```python
from build123d import *

# Parameters (mm, degrees)
SKETCH1_R           = 4.5
BOSS_EXTRUDE1_DEPTH = 8
SKETCH2_W           = 10
SKETCH2_H           = 25
BOSS_EXTRUDE2_DEPTH = 34.4
SKETCH5_W           = 10
SKETCH5_H           = 10
BOSS_EXTRUDE4_DEPTH = 8
SKETCH6_R           = 1.5
CUT_EXTRUDE1_DEPTH  = 15
SKETCH10_W          = 25
SKETCH10_H          = 32.5
BOSS_EXTRUDE6_DEPTH = 12
SKETCH12_W          = 12
SKETCH12_H          = 21.5
CUT_EXTRUDE3_DEPTH  = 21.5
SKETCH13_R          = 1
CUT_EXTRUDE4_DEPTH  = 10
SKETCH14_W          = 9
SKETCH14_H          = 13
CUT_EXTRUDE5_DEPTH  = 38.45
CUT_EXTRUDE6_REACH  = 59
SKETCH15_W          = 15
SKETCH15_H          = 20.5
SKETCH16_R          = 3
BOSS_EXTRUDE7_DEPTH = 5


with BuildPart() as part:
    # Sketch1 → Boss-Extrude1 (new body)
    with BuildSketch(Plane(origin=(0, 0, 0), x_dir=(1, 0, 0), z_dir=(0, 1, 0))):
        with BuildLine():
            Line((0, 0), (40, 0))
            ThreePointArc((40, 0), (43.535533906, 1.464466094), (45, 5))
            Line((45, 5), (45, 20))
            ThreePointArc((45, 20), (43.535533906, 23.535533906), (40, 25))
            Line((40, 25), (0, 25))
            Line((0, 25), (0, 0))
        make_face()
        with Locations((37.263316161, 12.5)):
            Circle(SKETCH1_R, mode=Mode.SUBTRACT)
    extrude(amount=BOSS_EXTRUDE1_DEPTH)

    # Sketch2 → Boss-Extrude2 (add)
    with BuildSketch(Plane(origin=(0, 8, 0), x_dir=(1, 0, 0), z_dir=(0, 1, 0))):
        with Locations((5, 12.5)):
            Rectangle(SKETCH2_W, SKETCH2_H)
    extrude(amount=BOSS_EXTRUDE2_DEPTH)

    # Sketch5 → Boss-Extrude4 (add)
    with BuildSketch(Plane(origin=(0, 42.4, 0), x_dir=(1, 0, 0), z_dir=(0, 1, 0))):
        with Locations((5, 12.5)):
            Rectangle(SKETCH5_W, SKETCH5_H)
    extrude(amount=BOSS_EXTRUDE4_DEPTH)

    # Sketch6 → Cut-Extrude1 (cut)
    with BuildSketch(Plane(origin=(0, 42.4, 0), x_dir=(1, 0, 0), z_dir=(0, 1, 0))):
        with Locations((5, 21.25)):
            Circle(SKETCH6_R)
        with Locations((5, 3.75)):
            Circle(SKETCH6_R)
    extrude(amount=-CUT_EXTRUDE1_DEPTH, mode=Mode.SUBTRACT)

    # Sketch10 → Boss-Extrude6 (add)
    with BuildSketch(Plane.ZY):
        with Locations((-12.5, 21.2)):
            Rectangle(SKETCH10_W, SKETCH10_H)
    extrude(amount=BOSS_EXTRUDE6_DEPTH)

    # Sketch12 → Cut-Extrude3 (cut)
    with BuildSketch(Plane(origin=(0, 0, -25), x_dir=(-1, 0, 0), z_dir=(0, 0, -1))):
        with Locations((3, 21.2)):
            Rectangle(SKETCH12_W, SKETCH12_H)
    extrude(amount=-CUT_EXTRUDE3_DEPTH, mode=Mode.SUBTRACT)

    # Sketch13 → Cut-Extrude4 (cut)
    with BuildSketch(Plane(origin=(0, 0, -25), x_dir=(-1, 0, 0), z_dir=(0, 0, -1))):
        with Locations((3, 35.2)):
            Circle(SKETCH13_R)
        with Locations((3, 7.2)):
            Circle(SKETCH13_R)
    extrude(amount=-CUT_EXTRUDE4_DEPTH, mode=Mode.SUBTRACT)

    # Sketch14 → Cut-Extrude5 (cut, through all)
    with BuildSketch(Plane(origin=(0, 37.45, 0), x_dir=(1, 0, 0), z_dir=(0, 1, 0))):
        with Locations((-4.5, 10.945919096)):
            Rectangle(SKETCH14_W, SKETCH14_H)
    extrude(amount=-CUT_EXTRUDE5_DEPTH, mode=Mode.SUBTRACT)

    # Sketch15 → Cut-Extrude6 (cut, up to next)
    with BuildSketch(Plane.ZY.offset(12), mode=Mode.PRIVATE) as cut_extrude6_sk1:
        with Locations((-12.5, 21.2)):
            Rectangle(SKETCH15_W, SKETCH15_H)
    cut_extrude6_tool1 = extrude(cut_extrude6_sk1.sketch, amount=-CUT_EXTRUDE6_REACH, mode=Mode.PRIVATE) & part.part
    add(cut_extrude6_tool1.solids().sort_by_distance((-12, 21.2, -12.5))[0], mode=Mode.SUBTRACT)

    # Sketch16 → Boss-Extrude7 (add)
    with BuildSketch(Plane.XY):
        with Locations((-3, 26.45)):
            Circle(SKETCH16_R)
    extrude(amount=BOSS_EXTRUDE7_DEPTH)


solid = part.part
```
Geometry: final body of the model. Coordinates: model frame, mm. A direction names the side the tool comes from. Coordinates: 2 decimals unless noted, no trailing zeros. Order: outer loops, then holes, each group sorted by start corner. A loop starts at its lowest first (then second) coordinate and runs counter-clockwise, first axis right, second up. Notation, with made-up numbers: (-4, 0) - (15, 0) arc R17 cw to (15, 10) - close; hole circle Ø3 at (77, 26). An arc over 180 degrees is marked (long way). Write each question's results on one line, items separated by ' | '.
1) Section C-C, the plane x = -3. Return loops of the section in (y, z), plus the area to 3 significant figures.
Results list:
outline: (4.95, -25) - (6.2, -25) - (6.2, -17.45) - (4.95, -17.45) - close; (4.95, -4.45) - (10.45, -4.45) - (10.45, -3.5) - (31.95, -3.5) - (31.95, -4.45) - (37.45, -4.45) - (37.45, 0) - (29.45, 0) - (29.45, 5) - (23.45, 5) - (23.45, 0) - (4.95, 0) - close; (8.2, -25) - (10.45, -25) - (10.45, -17.45) - (8.2, -17.45) - close; (31.95, -25) - (34.2, -25) - (34.2, -17.45) - (31.95, -17.45) - close; (36.2, -25) - (37.45, -25) - (37.45, -17.45) - (36.2, -17.45) - close | area: 207 mm^2
2) Section B-B, the plane y = 35.2. Return loops of the section in (x, z).
Results list:
outline: (-12, -25) - (-4, -25) - (-4, -17.45) - (-9, -17.45) - (-9, -4.45) - (0, -4.45) - (0, -17.45) - (-2, -17.45) - (-2, -25) - (10, -25) - (10, 0) - (-12, 0) - close; hole circle Ø3 at (5, -21.25); hole circle Ø3 at (5, -3.75)
3) Pin query (flat end, axial travel): pin 1 (6.5 mm diameter, centred on y = 21, z = -11, fed in from -X); pin 2 (6 mm diameter, centred on x = -4, z = -14.5, fed in from -Y); pin 3 (9 mm diameter, centred on x = 4, y = 45, fed in from +Z). Return the tip coordinate at first contact, or that it passes through.
Results list:
pin 1: x = 3 | pin 2: y = 4.95 | pin 3: z = 0
4) Section D-D, the plane y = 26.45. Return loops of the section in (x, z), plus the area to 3 significant figures.
Results list:
outline: (-12, -25) - (-9, -25) - (-9, -20) - (-12, -20) - close; (-12, -5) - (-9, -5) - (-9, -3.5) - (3, -3.5) - (3, -25) - (10, -25) - (10, 0) - (0, 0) - (0, 5) - (-6, 5) - (-6, 0) - (-12, 0) - close | area: 277 mm^2
5) Line query: line 1 (Z direction, x = 5, y = 35.5); line 2 (X direction, y = 33, z = -12); line 3 (X direction, y = 6, z = -10.5). Output: solid intervals per line, ascending. Write a range as from..to.
Results list:
line 1: -25..-22.75, -19.75..-5.25, -2.25..0 | line 2: -12..-9, 0..10 | line 3: -12..-9, 0..33.23, 41.29..45
6) Pull-direction query (X, two-part tool) for faces 1 (the flat face through (45, 4, -12)), 2 (the cylindrical face through (6.386, 35.005, -3.175)), 3 (the flat face through (8, 16, -25)); classes: pulls with the +X half, pulls with the -X half, needs draft (parallel to the pull), parting line crosses it, or undercut.
Results list:
face 1: pulls with the +X half | face 2: undercut | face 3: needs draft
7) Section A-A, the plane z = -12.5. Return loops of the section in (x, y).
Results list:
outline: (-12, 4.95) - (-9, 4.95) - (-9, 10.95) - (-12, 10.95) - close; (-12, 31.45) - (-9, 31.45) - (-9, 37.45) - (-12, 37.45) - close; (0, 0) - (32.76, 0) - (32.76, 8) - (10, 8) - (10, 50.4) - (0, 50.4) - (0, 31.95) - (3, 31.95) - (3, 10.45) - (0, 10.45) - close; (41.76, 0) - (45, 0) - (45, 8) - (41.76, 8) - close
8) Set-up query: faces 4 (the flat face through (-11, 21, -5)), 5 (the flat face through (5, 46, -7.5)), 6 (the flat face through (-5, 35, -4.446)), 7 (the flat face through (-3, 21, -3.5)). Return all of +Z, -Z, +X, -X, +Y, -Y with unobstructed straight access to the full face (end or side cutting, diameter ignored); none if empty.
Results list:
face 4: -X | face 5: +Z, +X, -X, +Y | face 6: +Y, -Y | face 7: -Z
